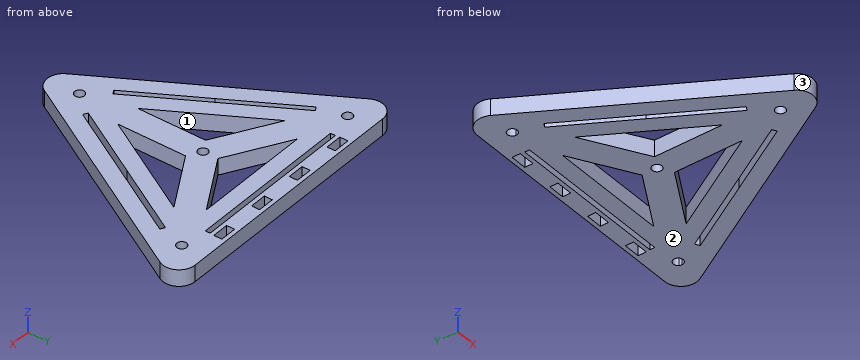
from build123d import *

# Parameters (mm, degrees)
F0_R     = 1.5
F1_DEPTH = 5.08
F2_R     = 5
F3_W     = 50
F3_H     = 1.5
F3_W_2   = 5.08
F3_H_2   = 2.5
F4_DEPTH = 25


with BuildPart() as f1:
    # F0 (on Top) → F1 (new body)
    with BuildSketch(Plane.XY):
        Polygon((0, 78.118305), (-46.115853, 78.118305), (0, -1.756695), (46.115853, 78.118305), align=None)
        with Locations((0, 13.243305)):
            Circle(F0_R, mode=Mode.SUBTRACT)
        Polygon((-18.197268, 66.618305), (0, 66.618305), (18.197268, 66.618305), (26.197268, 66.618305), (22.197268, 59.690101), (4, 28.171508), (0, 21.243305), (-4, 28.171508), (-22.197268, 59.690101), (-26.197268, 66.618305), align=None, mode=Mode.SUBTRACT)
        with BuildLine():
            ThreePointArc((-34.42451, 71.368305), (-32.737243, 72.067193), (-31.625472, 70.618305))
            ThreePointArc((-31.625472, 70.618305), (-33.5137, 69.169416), (-34.42451, 71.368305))
        make_face(mode=Mode.SUBTRACT)
        with BuildLine():
            ThreePointArc((34.625472, 70.618305), (31.676583, 70.230076), (34.42451, 71.368305))
            ThreePointArc((34.42451, 71.368305), (34.57436, 71.006533), (34.625472, 70.618305))
        make_face(mode=Mode.SUBTRACT)
        Polygon((26.197268, 66.618305), (18.197268, 66.618305), (0, 56.112107), (-18.197268, 66.618305), (-26.197268, 66.618305), (-22.197268, 59.690101), (-4, 49.183903), (-4, 28.171508), (0, 21.243305), (4, 28.171508), (4, 49.183903), (22.197268, 59.690101), align=None)
        with Locations((0, 51.493305)):
            Circle(F0_R, mode=Mode.SUBTRACT)
    extrude(amount=F1_DEPTH)

    # F2
    f2_edges = [f1.edges().sort_by_distance(p)[0] for p in [
        (-46.115853, 78.118305, 2.54),
        (0, -1.756695, 2.54),
        (46.115853, 78.118305, 2.54),
    ]]
    fillet(f2_edges, radius=F2_R)

    # F3 (on face) → F4 (cut)
    with BuildSketch(Plane.XY.offset(5.08)):
        with Locations((0, 72.368305)):
            Rectangle(F3_W, F3_H)
        Polygon((-6.227799, 19.030169), (-5.57828, 19.405169), (-4.928761, 19.780169), (-17.428761, 41.430805), (-29.928761, 63.08144), (-30.57828, 62.70644), (-31.227799, 62.33144), (-18.727799, 40.680805), align=None)
        Polygon((30.57828, 62.70644), (29.928761, 63.08144), (17.428761, 41.430805), (4.928761, 19.780169), (5.57828, 19.405169), (6.227799, 19.030169), (18.727799, 40.680805), (31.227799, 62.33144), align=None)
        Polygon((10.08, 76.868305), (5, 76.868305), (5, 75.618305), (5, 74.368305), (10.08, 74.368305), align=None)
        with Locations((22.62, 75.618305)):
            Rectangle(F3_W_2, F3_H_2)
        with Locations((-22.62, 75.618305)):
            Rectangle(F3_W_2, F3_H_2)
        with Locations((-7.54, 75.618305)):
            Rectangle(F3_W_2, F3_H_2)
    extrude(amount=-F4_DEPTH, mode=Mode.SUBTRACT)


solid = f1.part
Source: CAD feature listing. Evaluate the final solid. Frame: model axes, mm. Face numbers are marked on the shaded views. Coordinates: 2 decimals unless noted, no trailing zeros. Loops run counter-clockwise (first coordinate to the right, second up) from the corner with the lowest first, then second, coordinate; pieces in that order, holes last. Notation, with made-up numbers: M -8,36.5 L 40,36.5 A11 ccw 40,46.5 Z; hole C 53.5,19 d8. An arc over 180 degrees is marked long. Answer in a Markdown table with one row per item.
Q1. Draft query along Y for the marked faces 1, 2 and 3. Return one class per face: pulls with the +Y half, pulls with the -Y half, needs draft (parallel to the pull), parting line crosses it, or undercut.
Answers below:
| item | result |
|---|---|
| face 1 | undercut |
| face 2 | needs draft |
| face 3 | pulls with the -Y half |
Q2. First-contact query: pin 1 (2 mm diameter, centred on y = 75, z = 3, fed in from -X); pin 2 (0.8 mm diameter, centred on y = 72.5, z = 3, fed in from -X); pin 3 (1.5 mm diameter, centred on x = 21.5, z = 3.5, fed in from -Y); pin 4 (2.5 mm diameter, centred on x = 0, y = 13.24, fed in from -Z). Flat tips, straight axial feed; report the tip coordinate or a pass-through.
Answers below:
| item | result |
|---|---|
| pin 1 | stops at x = -42.38 |
| pin 2 | stops at x = -42.45 |
| pin 3 | stops at y = 34.18 |
| pin 4 | passes through |
Q3. Ray query, probe 1 along X at (y, z) = (26.5, 4.5); probe 2 along X at (y, z) = (28.5, 0.3); probe 3 along X at (y, z) = (23, 4.55). Return the intervals inside material, ascending. Write a range as from..to.
Answers below:
| item | result |
|---|---|
| probe 1 | x = -16.31..-10.54, -8.81..8.81, 10.54..16.31 |
| probe 2 | x = -17.47..-11.7, -9.96..-4.19, -4..4, 4.19..9.96, 11.7..17.47 |
| probe 3 | x = -14.29..-8.52, -6.79..6.79, 8.52..14.29 |
Q4. Section A-A on y = 25.5. Return the cut outline in (x, z).
Answers below:
| item | result |
|---|---|
| outline | M -15.74,0 L -9.96,0 L -9.96,5.08 L -15.74,5.08 Z; M -8.23,0 L 8.23,0 L 8.23,5.08 L -8.23,5.08 Z; M 9.96,0 L 15.74,0 L 15.74,5.08 L 9.96,5.08 Z |
Q5. Section B-B on x = 21. Return the cut outline in (y, z).
Answers below:
| item | result |
|---|---|
| outline | M 34.62,0 L 44.62,0 L 44.62,5.08 L 34.62,5.08 Z; M 47.62,0 L 57.62,0 L 57.62,5.08 L 47.62,5.08 Z; M 59,0 L 71.62,0 L 71.62,5.08 L 59,5.08 Z; M 73.12,0 L 74.37,0 L 74.37,5.08 L 73.12,5.08 Z; M 76.87,0 L 78.12,0 L 78.12,5.08 L 76.87,5.08 Z |
Q6. Section C-C on z = 3. State how many separate pieces and enclosed holes the cut face has, plus the area to 3 significant figures.
Answers below:
| item | result |
|---|---|
| separate pieces | 1 |
| enclosed holes | 14 |
| area | 2,750 mm^2 |
Q7. Section D-D on x = 36.5. Return the cut outline in (y, z), plus the area to 3 significant figures.
Answers below:
| item | result |
|---|---|
| outline | M 61.46,0 L 78.12,0 L 78.12,5.08 L 61.46,5.08 Z |
| area | 84.6 mm^2 |
